```python
from build123d import *

# Parameters (mm, degrees)
SKETCH2_W          = 1
SKETCH2_H          = 2
SKETCH3_R          = 3
CUT_EXTRUDE1_DEPTH = 16


with BuildPart() as part:
    # Sketch1 → Revolve-Thin1 (revolve)
    with BuildSketch(Plane.XY):
        with BuildLine():
            Line((15, 0), (15, -2))
            Line((15, -2), (1.349281284, -14.47629266))
            ThreePointArc((1.349281284, -14.47629266), (0.723676268, -14.864481874), (0, -15))
            Line((0, -15), (0, -14.5))
            ThreePointArc((0, -14.5), (0.542757201, -14.398361406), (1.011960963, -14.107219495))
            Line((1.011960963, -14.107219495), (14.5, -1.779610529))
            Line((14.5, -1.779610529), (14.5, 0))
            Line((14.5, 0), (15, 0))
        make_face()
    revolve(axis=Axis((0, 0, 0), (0, -1, 0)))

    # Sketch2 → Revolve1 (revolve)
    with BuildSketch(Plane.XY):
        with Locations((-15.5, -1)):
            Rectangle(SKETCH2_W, SKETCH2_H)
    revolve(axis=Axis((0, 0, 0), (0, -1, 0)))

    # Sketch3 → Cut-Extrude1 (cut, through all)
    with BuildSketch(Plane(origin=(0, 0, 0), x_dir=(-1, 0, 0), z_dir=(0, 1, 0))):
        Circle(SKETCH3_R)
    extrude(amount=-CUT_EXTRUDE1_DEPTH, mode=Mode.SUBTRACT)


solid = part.part
```
Model file for the job. Use its own axes, mm. Give positions to 0.01 mm unless a question says otherwise; leave off trailing zeros. Loops run counter-clockwise (first coordinate to the right, second up) from the corner with the lowest first, then second, coordinate; pieces in that order, holes last. Notation, with made-up numbers: M 31.5,22.5 L 75.5,22.5 A23 ccw 75.5,49.5 Z; hole C 52,75.25 d8. An arc over 180 degrees is marked long. Use one line per item in the form item = value.
Item 1: Slice it at A-A on z = 0. List the corners of the cut face in (x, y), and give its area (3 significant figures).
Filled in:
outline = M -16,-2 L -15,-2 L -3,-12.97 L -3,-12.29 L -14.5,-1.78 L -14.5,0 L -16,0 Z; M 3,-12.97 L 15,-2 L 16,-2 L 16,0 L 14.5,0 L 14.5,-1.78 L 3,-12.29 Z
area = 21.8 mm^2
Item 2: Two-plate mould, pull along X, no slides. Class faces 1 (the cylindrical face through (3.47, -0.99, 15.62)), 2 (the flat face through (3.6, 0, -14.3)), 3 (the cylindrical face through (6.691, -0.877, -12.864)): released by +X, released by -X, zero draft, split by the parting line, or undercut.
Filled in:
face_1 = split by the parting line
face_2 = zero draft
face_3 = undercut
Item 3: Slice it at C-C on y = -0.75. List the corners of the cut face in (x, z).
Filled in:
outline = C 0,0 d32; hole C 0,0 d29
Item 4: Flat gauge pins, fed straight in: pin 1 Ø4 at (x, z) = (1.5, -1) entering from +Y; pin 2 Ø6 at (x, y) = (-5.5, -8.5) entering from -Z; pin 3 Ø1.5 at (x, y) = (4.5, -4.5) entering from -Z; pin 4 Ø3 at (x, z) = (12, -9) entering from +Y. Where does each tip first touch, or does it go through?
Filled in:
pin_1 = -11.56
pin_2 = -10.02
pin_3 = -12.33
pin_4 = 0
Item 5: Drill centre lines: L1, parallel to Z at x = 0, y = -1.2; L2, parallel to X at y = -11.25, z = -2; L3, parallel to Y at x = -13.5, z = -7. Where is each one in solid material? Low to high.
Filled in:
L1 = -16 to -14.5, 14.5 to 16
L2 = -4.45 to -3.62, 3.62 to 4.45
L3 = -2 to 0
Item 6: Slice it at D-D on y = -5. List the corners of the cut face in (x, z).
Filled in:
outline = C 0,0 d23.44; hole C 0,0 d21.95
Item 7: Slice it at B-B on x = 0. List the corners of the cut face in (y, z), and give its area (3 significant figures).
Filled in:
outline = M -12.97,-3 L -2,-15 L -2,-16 L 0,-16 L 0,-14.5 L -1.78,-14.5 L -12.29,-3 Z; M -12.97,3 L -12.29,3 L -1.78,14.5 L 0,14.5 L 0,16 L -2,16 L -2,15 Z
area = 21.8 mm^2
